Build history of the part. All positions in model axes, mm. Round coordinates to 2 decimals unless told otherwise and drop trailing zeros. One line per question, with ' | ' between items.
from build123d import *

# Parameters (mm, degrees)
F0_W     = 50.984893
F0_H     = 2.100501
F0_W_2   = 50.602986
F0_H_2   = 2.482414
F0_W_3   = 51.175848
F0_H_3   = 2.86432
F0_H_4   = 3.246229
F0_W_4   = 50.412029
F0_W_5   = 50.221075
F0_W_6   = 50.030118
F0_H_5   = 2.673368
F0_W_7   = 49.839167
F0_H_6   = 2.864324
F1_DEPTH = 12.7


with BuildPart() as f1:
    # F0 (on Front) → F1 (new body)
    with BuildSketch(Plane.XZ):
        Polygon((-48.025098, -41.532639), (-48.025098, -55.854235), (47.834139, -55.854235), (47.834139, -41.532639), (12.698486, -41.532639), (12.698486, -38.859274), (47.834139, -38.859274), (47.834139, -29.120585), (12.698486, -29.120585), (12.698486, -26.06531), (47.834139, -26.06531), (47.834139, -16.326623), (12.125621, -16.326623), (12.125621, -12.889439), (47.834139, -12.889439), (47.834139, -3.91457), (12.125621, -3.91457), (12.125621, -1.43216), (47.834139, -1.43216), (47.834139, 8.497482), (12.125621, 8.497482), (12.125621, 11.552757), (47.834139, 11.552757), (47.834139, 20.71858), (12.125621, 20.71858), (12.125621, 23.5829), (47.834139, 23.5829), (47.834139, 31.030132), (12.125621, 31.030132), (12.125621, 33.703495), (47.834139, 33.703495), (47.834139, 66.356741), (-48.025098, 66.356741), (-48.025098, 33.703495), (-11.361802, 33.703495), (-11.361802, 30.457268), (-48.025098, 30.457268), (-48.025098, 22.819081), (-11.361802, 22.819081), (-11.361802, 19.763807), (-48.025098, 19.763807), (-48.025098, 10.979893), (-11.361802, 10.979893), (-11.361802, 7.924618), (-48.025098, 7.924618), (-48.025098, -1.43216), (-11.361802, -1.43216), (-11.361802, -4.29648), (-48.025098, -4.29648), (-48.025098, -12.889439), (-11.361802, -12.889439), (-11.361802, -16.326623), (-48.025098, -16.326623), (-48.025098, -26.06531), (-11.170847, -26.06531), (-11.170847, -29.120585), (-48.025098, -29.120585), (-48.025098, -38.859274), (-11.170847, -38.859274), (-11.170847, -41.532639), align=None)
        with Locations((2.291455, -46.783892)):
            Rectangle(F0_W, F0_H, mode=Mode.SUBTRACT)
        with Locations((2.100502, -33.989929)):
            Rectangle(F0_W_2, F0_H_2, mode=Mode.SUBTRACT)
        with Locations((2.386933, -21.195967)):
            Rectangle(F0_W_3, F0_H_3, mode=Mode.SUBTRACT)
        with Locations((2.291455, -8.592959)):
            Rectangle(F0_W, F0_H_4, mode=Mode.SUBTRACT)
        with Locations((2.005024, 3.437183)):
            Rectangle(F0_W_4, F0_H_4, mode=Mode.SUBTRACT)
        with Locations((1.909546, 15.276373)):
            Rectangle(F0_W_5, F0_H_4, mode=Mode.SUBTRACT)
        with Locations((1.814068, 27.401994)):
            Rectangle(F0_W_6, F0_H_5, mode=Mode.SUBTRACT)
        with Locations((1.718592, 37.236158)):
            Rectangle(F0_W_7, F0_H_6, mode=Mode.SUBTRACT)
    extrude(amount=F1_DEPTH)


solid = f1.part
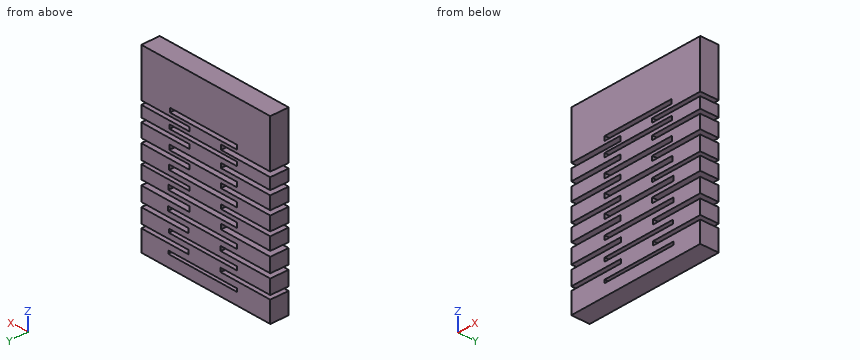
(1) Wall check: line 1 (X direction, y = -7.75, z = -10); line 2 (X direction, y = -9.5, z = -26.5). Give the ranges that are in metal, low to high. Write a range as from..to.
Calculated:
line 1: -48.03..-23.2, 27.78..47.83 | line 2: -11.17..12.7
(2) Drop flat-ended pins along their axis: pin 1 (1 mm diameter, centred on y = -8, z = -14, fed in from +X); pin 2 (1 mm diameter, centred on y = -7.5, z = -14, fed in from -X). Give the stop position or say it passes through.
Calculated:
pin 1: x = 12.13 | pin 2: x = -11.36
(3) Slice it at A-A (x = 33). State how many separate pieces and enclosed holes the cut face has, then the cut area to 3 significant figures.
Calculated:
separate pieces: 8 | enclosed holes: 0 | area: 1,300 mm2
